from build123d import *

# Parameters (mm, degrees)
SKETCH1_R           = 25
BOSS_EXTRUDE1_DEPTH = 3
SKETCH3_R           = 1.7
CUT_EXTRUDE1_DEPTH  = 44.528946063


with BuildPart() as part:
    # Sketch1 → Boss-Extrude1 (new body)
    with BuildSketch(Plane(origin=(0, 0, 0), x_dir=(1, 0, 0), z_dir=(0, 1, 0))):
        with Locations(Location((0, 0, 0), (0, 0, 270))):
            Circle(SKETCH1_R)
    extrude(amount=BOSS_EXTRUDE1_DEPTH)

    # Sketch2 → Revolve1 (revolve)
    with BuildSketch(Plane(origin=(0, 0, 0), x_dir=(0, 0, -1), z_dir=(1, 0, 0)), mode=Mode.PRIVATE) as revolve1_sk:
        Polygon((-8, 3), (-2, 25.392304845), (0, 25.392304845), (0, 3), align=None)
    revolve(revolve1_sk.sketch.rotate(Axis((0, 0, 0), (0, 1, 0)), 180), axis=Axis((0, 0, 0), (0, 1, 0)))

    # Sketch3 → Cut-Extrude1 (cut, through all)
    with BuildSketch(Plane(origin=(0, 25.392304845, 0), x_dir=(1, 0, 0), z_dir=(0, 1, 0))):
        with Locations(Location((0, 0, 0), (0, 0, 270))):
            Circle(SKETCH3_R)
    extrude(amount=-CUT_EXTRUDE1_DEPTH, mode=Mode.SUBTRACT)


solid = part.part
Model file for the job. Use its own axes, mm. Give positions to 0.01 mm unless a question says otherwise; leave off trailing zeros. Write each loop counter-clockwise with the first axis right and the second up, starting at its lowest first coordinate (ties: lowest second). Pieces come first, ordered by that corner, then holes. Notation, with made-up numbers: M 46,40.25 L 61,40.25 A23 ccw 61,58.25 Z; hole C 69,84.5 d9. An arc over 180 degrees is marked long. One line per item, written item: value. Start each with the question number.
Q1. Probe probe 1 along Y at (x, z) = (-14.5, 8); probe 2 along Z at (x, y) = (-1, 9.5); probe 3 along X at (y, z) = (13, 0). List the from-to ranges inside material, lowest first. Write a range as [from, to].
Q2. Saw through at A-A, the plane x = 0. Write the cut outline in (y, z).
Q3. Saw through at B-B, the plane z = 0. Write the cut outline in (x, y).
Q4. Saw through at D-D, the plane x = 15. Write the cut outline in (y, z).
Q5. Two-plate mould, pull along Z, no slides. Class faces 1 (the cylindrical face through (7.509, 1.479, 23.846)), 2 (the flat face through (6, 3, -6)), 3 (the cylindrical face through (-1.66, 12.87, -0.37)): +Z half, -Z half, draft (parallel to the pull), parting line (faces both ways), or undercut.
Q6. Saw through at C-C, the plane y = 9.5. Write the cut outline in (x, z).
Q7. Drop flat-ended pins along their axis: pin 1 Ø5 at (x, z) = (8, -18) entering from +Y; pin 2 Ø5 at (y, z) = (11, -3) entering from -X; pin 3 Ø12 at (y, z) = (18.5, 8.5) entering from -X. Give the stop position or say it passes through.
Output values:
1. probe 1: y = [0, 3]
1. probe 2: z = [-6.18, -1.37], [1.37, 6.18]
1. probe 3: x = [-5.32, -1.7], [1.7, 5.32]
2. outline: M 0,-25 L 3,-25 L 3,-8 L 25.39,-2 L 25.39,-1.7 L 0,-1.7 Z; M 0,1.7 L 25.39,1.7 L 25.39,2 L 3,8 L 3,25 L 0,25 Z
3. outline: M -25,0 L -1.7,0 L -1.7,25.39 L -2,25.39 L -8,3 L -25,3 Z; M 1.7,0 L 25,0 L 25,3 L 8,3 L 2,25.39 L 1.7,25.39 Z
4. outline: M 0,-20 L 3,-20 L 3,20 L 0,20 Z
5. face 1: parting line
5. face 2: draft
5. face 3: undercut
6. outline: C 0,0 d12.52; hole C 0,0 d3.4
7. pin 1: stops at y = 3
7. pin 2: stops at x = -6.22
7. pin 3: stops at x = -3.34
